For this review, take the finished solid that the model builds, in its own axes (mm). A direction names the side the tool comes from. Coordinates: 2 decimals unless noted, no trailing zeros. Loops run counter-clockwise (first coordinate to the right, second up) from the corner with the lowest first, then second, coordinate; pieces in that order, holes last. Notation, with made-up numbers: M 88.5,44.25 L 110.5,44.25 A5 cw 110.5,53.25 Z; hole C 25.5,5.5 d2. An arc over 180 degrees is marked long. Answer as a JSON object with one key per item and string values. Group by question number.
Item 1: Tool access review of faces 1 (the face through (-99.006, -379.227, -177.548)), 2 (the face through (-15, 31, 131.5)): name each direction out of +Z, -Z, +X, -X, +Y, -Y from which nothing blocks a thin tool from reaching the whole face with its end or side.
Item 2: Wall thickness on L1, parallel to Y at x = -19.5, z = -198; L2, parallel to Z at x = -233, y = 231.5; L3, parallel to X at y = 236, z = -84: over which ranges is each line inside the solid? List them lowest first. Write a range as from..to.
Item 3: Add section A-A (z = -162.5). State the section outline as (x, y) points, then the cut area to 3 significant figures.
Item 4: Add section B-B (z = 26.5). State the section outline as (x, y) points.
Item 5: Insertion check: pin 1 (2 mm diameter, centred on x = 219.5, z = -159, fed in from -Y); pin 2 (12 mm diameter, centred on y = -288.5, z = 20, fed in from -X); pin 3 (12 mm diameter, centred on x = 298.5, y = -239.5, fed in from -Z). Each pin has a flat end and moves straight along its axis. Give the tip position at first contact, or say it passes through.
Item 6: Mouldability with a two-part tool opening along X and no side actions: class faces 3 (the face through (-313.34, -207.91, 148.24)), 4 (the face through (-363, 251, -274.646)), 5 (the face through (402.1, 154.84, -177.55)) as +X half, -X half, draft (parallel to the pull), parting line (faces both ways), or undercut.
from build123d import *

# Parameters (mm, degrees)
SKETCH1_R           = 33.167751503
SKETCH1_R_2         = 31.877533848
BOSS_EXTRUDE1_DEPTH = 14.732
SKETCH4_R           = 29.484523805
SKETCH1_3_R         = 33.167751503
SKETCH5_R           = 29.484523805
CUT_EXTRUDE1_DEPTH  = 2.54
SCALE1_SCALE        = 13


with BuildPart() as part:
    # Sketch1 → Boss-Extrude1 (new body)
    with BuildSketch(Plane.XY):
        with Locations((-9.170341316, 25.326095841)):
            Circle(SKETCH1_R)
        with Locations((-9.170341316, 25.326095841)):
            Circle(SKETCH1_R_2, mode=Mode.SUBTRACT)
    extrude(amount=-BOSS_EXTRUDE1_DEPTH)

    # Sketch4 → Loft1 section 0
    with BuildSketch(Plane.XY.offset(19.05)):
        with Locations((-9.170341316, 25.326095841)):
            Circle(SKETCH4_R)
    # Sketch1<3> → Loft1 section 1
    with BuildSketch(Plane.XY):
        with Locations((-9.170341316, 25.326095841)):
            Circle(SKETCH1_3_R)
    loft()

    # Sketch5 → Cut-Extrude1 (cut)
    with BuildSketch(Plane.XY.offset(19.05)):
        with Locations((-9.170341316, 25.326095841)):
            Circle(SKETCH5_R)
    extrude(amount=-CUT_EXTRUDE1_DEPTH, mode=Mode.SUBTRACT)


with BuildPart() as part_1:
    # Scale1: scaled about (-9.170341316, 25.326095841, 6.927517959)
    add(part.part.scale(SCALE1_SCALE).moved(Location((110.044095792, -303.913150092, -83.130215508))))


solid = part_1.part
From the geometry:
{
 "1": {"face 1": "-Z", "face 2": "+Z"},
 "2": {"L1": "y = -405.73..-388.95, 439.61..456.38", "L2": "z = -83.13..131.5", "L3": "x = -385.38..-366.03, 347.69..367.04"},
 "3": {"outline": "C -9.17,25.33 d862.36; hole C -9.17,25.33 d828.82", "area": "44,600 mm²"},
 "4": {"outline": "C -9.17,25.33 d819.97"},
 "5": {"pin 1": "stops at y = -340.85", "pin 2": "stops at x = -282.09", "pin 3": "stops at z = -83.13"},
 "6": {"face 3": "undercut", "face 4": "draft", "face 5": "parting line"}
}
